from build123d import *

# Parameters (mm, degrees)
F1_DEPTH = 25.4
F0_W     = 16.073438
F0_H     = 4.7625
F3_R     = 2.182813
F4_DEPTH = 2.9718
F6_DEPTH = 19.051


with BuildPart() as f1:
    # F0 (on Front) → F1 (new body, symmetric)
    with BuildSketch(Plane.XZ):
        Polygon((-6.737426, 63.6778), (-9.713988, 63.6778), (-9.713988, 0), (9.336012, 0), (9.336012, 2.9718), (-6.737426, 2.9718), (-6.737426, 48.8315), (-6.737426, 53.594), (-6.737426, 58.3565), align=None)
    extrude(amount=F1_DEPTH, both=True)

    # F0 (on Front) → F2 (revolve)
    with BuildSketch(Plane.XZ):
        with Locations((1.299293, 55.97525)):
            Rectangle(F0_W, F0_H)
    revolve(axis=Axis((1.299293, 0, 53.594), (-1, 0, 0)))

    # F3 (on face) → F4 (cut, through all)
    with BuildSketch(Plane.XY.offset(2.9718)):
        with Locations((1.400099, 15.977813)):
            Circle(F3_R)
        with Locations((1.400099, -15.977813)):
            Circle(F3_R)
    extrude(amount=-F4_DEPTH, mode=Mode.SUBTRACT)

    # F5 (on face) → F6 (cut, through all)
    with BuildSketch(Plane(origin=(-9.713988, 0, 0), x_dir=(0, -1, 0), z_dir=(-1, 0, 0))):
        Polygon((25.4, 63.6778), (10.33, 63.6778), (25.4, 2.91), align=None)
        Polygon((-25.4, 2.91), (-10.33, 63.6778), (-25.4, 63.6778), align=None)
    extrude(amount=-F6_DEPTH, mode=Mode.SUBTRACT)


solid = f1.part
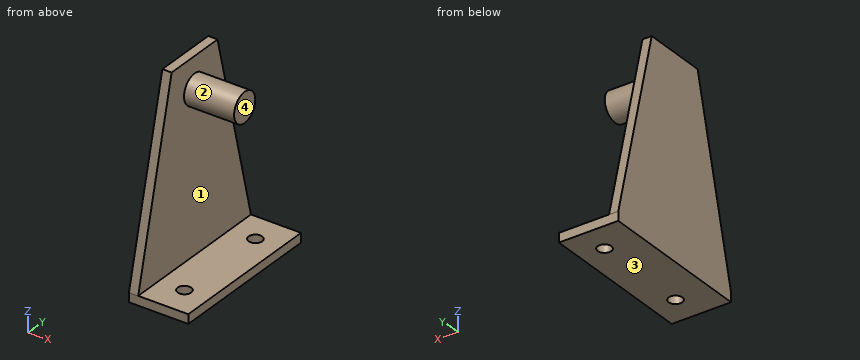
Part model, mm, in its own coordinate system. Face numbers are marked on the shaded views. Give positions to 0.01 mm unless a question says otherwise; leave off trailing zeros. Order: outer loops, then holes, each group sorted by start corner. A loop starts at its lowest first (then second) coordinate and runs counter-clockwise, first axis right, second up. Notation, with made-up numbers: (27, 89) - (48, 89) arc R28 ccw to (48, 120) - close; hole circle Ø3 at (-33.75, 44). An arc over 180 degrees is marked (long way). One line per question, with ' | ' between items.
1. Band-saw the part on D-D on z = 51. List the corners of the cut face in (x, y).
Filled in:
outline: (-9.71, -13.47) - (-6.74, -13.47) - (-6.74, -3.99) - (9.34, -3.99) - (9.34, 3.99) - (-6.74, 3.99) - (-6.74, 13.47) - (-9.71, 13.47) - close
2. Band-saw the part on B-B on y = 0. List the corners of the cut face in (x, z).
Filled in:
outline: (-9.71, 0) - (9.34, 0) - (9.34, 2.97) - (-6.74, 2.97) - (-6.74, 48.83) - (9.34, 48.83) - (9.34, 58.36) - (-6.74, 58.36) - (-6.74, 63.68) - (-9.71, 63.68) - close
3. Drill centre lines: probe 1 along X at (y, z) = (13.5, 8.5); probe 2 along Z at (x, y) = (7, 20); probe 3 along Z at (x, y) = (-2.25, 4). Where is each one in solid material? Low to high.
Filled in:
probe 1: -9.71 to -6.74 | probe 2: 0 to 2.97 | probe 3: 0 to 2.97, 51.01 to 56.18
4. Drop flat-ended pins along their axis: P1, Ø10, axis at x = -5.5, z = 41.5, coming from the -Y side; P2, Ø6, axis at y = 12.5, z = 9, coming from the +X side; P3, Ø1.5, axis at x = 7.5, z = 50.5, coming from the -Y side; P4, Ø8, axis at x = 1.5, y = -4, coming from the -Z side. Give the stop position or say it passes through.
Filled in:
P1: y = -17.03 | P2: x = -6.74 | P3: y = -4.15 | P4: z = 0
5. Pull direction Z, two halves, no side cores. Call the marked faces 1, 2, 3 and 4: +Z half, -Z half, draft (parallel to the pull), parting line (faces both ways), or undercut.
Filled in:
face 1: undercut | face 2: undercut | face 3: -Z half | face 4: draft
6. Band-saw the part on C-C on x = 0.5. Give the number of separate pieces and of enclosed holes in the cut face, then the cut area to 3 significant figures.
Filled in:
separate pieces: 4 | enclosed holes: 0 | area: 199 mm²
